```python
from build123d import *

# Parameters (mm, degrees)
BOSS_EXTRUDE1_DEPTH = 19
SKETCH2_W           = 32
SKETCH2_H           = 55
CUT_EXTRUDE1_DEPTH  = 45
SKETCH3_W           = 32
SKETCH3_H           = 22.717187721
CUT_EXTRUDE2_DEPTH  = 12
SKETCH4_R           = 4.5
CUT_EXTRUDE3_DEPTH  = 39
CUT_EXTRUDE4_REACH  = 71
SKETCH5_R           = 5.75
FILLET1_R           = 3


with BuildPart() as part:
    # Sketch1 → Boss-Extrude1 (new body, symmetric)
    with BuildSketch(Plane(origin=(0, 0, 0), x_dir=(0, 0, -1), z_dir=(1, 0, 0))):
        with BuildLine():
            Line((-11, 0), (-11, 58))
            Line((-11, 58), (33, 58))
            Line((33, 58), (10.326710033, -3.789335019))
            ThreePointArc((10.326710033, -3.789335019), (-1.924342697, -10.830369577), (-11, 0))
        make_face()
    extrude(amount=BOSS_EXTRUDE1_DEPTH, both=True)

    # Sketch2 → Cut-Extrude1 (cut, through all)
    with BuildSketch(Plane.XY.offset(11)):
        with Locations((0, 27.5)):
            Rectangle(SKETCH2_W, SKETCH2_H)
    extrude(amount=-CUT_EXTRUDE1_DEPTH, mode=Mode.SUBTRACT)

    # Sketch3 → Cut-Extrude2 (cut, through all)
    with BuildSketch(Plane(origin=(0, 0, 0), x_dir=(1, 0, 0), z_dir=(0, 1, 0))):
        with Locations((0, 0.358593861)):
            Rectangle(SKETCH3_W, SKETCH3_H)
    extrude(amount=-CUT_EXTRUDE2_DEPTH, mode=Mode.SUBTRACT)

    # Sketch4 → Cut-Extrude3 (cut, through all)
    with BuildSketch(Plane.ZY.offset(19)):
        Circle(SKETCH4_R)
    extrude(amount=-CUT_EXTRUDE3_DEPTH, mode=Mode.SUBTRACT)

    # Sketch5 → Cut-Extrude4 (cut, up to next)
    with BuildSketch(Plane(origin=(0, 58, 0), x_dir=(1, 0, 0), z_dir=(0, 1, 0)), mode=Mode.PRIVATE) as cut_extrude4_sk1:
        with Locations((0, 11)):
            Circle(SKETCH5_R)
    cut_extrude4_tool1 = extrude(cut_extrude4_sk1.sketch, amount=-CUT_EXTRUDE4_REACH, mode=Mode.PRIVATE) & part.part
    add(cut_extrude4_tool1.solids().sort_by_distance((0, 58, -11))[0], mode=Mode.SUBTRACT)

    # Fillet1
    fillet1_edges = [part.edges().sort_by_distance(p)[0] for p in [
        (19, 58, -11),
        (-19, 58, -11),
    ]]
    fillet(fillet1_edges, radius=FILLET1_R)


solid = part.part
```
The model under review builds one solid part; all positions refer to its coordinate system, in mm. A direction names the side the tool comes from. Round coordinates to 2 decimals unless told otherwise and drop trailing zeros. Order: outer loops, then holes, each group sorted by start corner. A loop starts at its lowest first (then second) coordinate and runs counter-clockwise, first axis right, second up. Notation, with made-up numbers: (49, -15) -> (86, -15) arc R16 ccw to (86, 5) -> close; hole circle Ø2 at (9.25, 81). An arc over 180 degrees is marked (long way). One line per item, written item: value. Start each with the question number.
Q1. Take a section at A-A (x = 0). Write out the cut boundary in (y, z), and give its area (3 significant figures).
Q2. Machinability: for faces 4 (the face through (4, 58, -6)), 5 (the face through (-4, 55, -5)), which of the approach directions +Z, -Z, +X, -X, +Y, -Y give a long, thin tool a straight path to every point of the face, cutting with its end or side? Answer none if there is none.
Q3. Mouldability with a two-part tool opening along X and no side actions: class faces 1 (the face through (18.14, 57.1, -11.31)), 2 (the face through (16, 29, -5)), 3 (the face through (17.521, -10.866, 1.712)) as released by +X, released by -X, zero draft, split by the parting line, or undercut.
Q4. Take a section at B-B (z = 0). Write out the cut boundary in (x, y).
Q5. Take a section at C-C (y = 16.5). Write out the cut boundary in (x, z).
Q6. Wall thickness on line 1 (X direction, y = 31, z = -9); line 2 (Y direction, x = -6, z = -3.5); line 3 (X direction, y = 55.7, z = -11): over which ranges is each line inside the solid? List them lowest first.
Q7. Clearance check with flat-ended pins moving along their axes: pin 1 Ø2 at (x, z) = (3.5, -28) entering from -Y; pin 2 Ø10 at (x, z) = (15, 6.5) entering from -Y. State where each tip first meets the part, or that it passes through.
Q8. Take a section at D-D (z = -29). Write out the cut boundary in (x, y), and give its area (3 significant figures).
Reported:
1. outline: (55, -31.9) -> (58, -33) -> (58, -16.75) -> (55, -16.75) -> close; (55, -5.25) -> (58, -5.25) -> (58, 11) -> (55, 11) -> close
1. area: 95.8 mm2
2. face 4: +Z, -Z, +X, -X, +Y
2. face 5: +Z, -Z, -Y
3. face 1: released by +X
3. face 2: undercut
3. face 3: zero draft
4. outline: (-19, -11) -> (-16, -11) -> (-16, -4.5) -> (-19, -4.5) -> close; (-19, 4.5) -> (-16, 4.5) -> (-16, 55) -> (16, 55) -> (16, 4.5) -> (19, 4.5) -> (19, 55) arc R3 ccw to (16, 58) -> (-16, 58) arc R3 ccw to (-19, 55) -> close; (16, -11) -> (19, -11) -> (19, -4.5) -> (16, -4.5) -> close
5. outline: (-19, -17.77) -> (-16, -17.77) -> (-16, 11) -> (-19, 11) -> close; (16, -17.77) -> (19, -17.77) -> (19, 11) -> (16, 11) -> close
6. line 1: x = -19 to -16, 16 to 19
6. line 2: y = 55 to 58
6. line 3: x = -18.92 to -5.75, 5.75 to 18.92
7. pin 1: stops at y = 55
7. pin 2: stops at y = -10.88
8. outline: (-19, 47.1) -> (-16, 47.1) -> (-16, 55) -> (16, 55) -> (16, 47.1) -> (19, 47.1) -> (19, 55) arc R3 ccw to (16, 58) -> (-16, 58) arc R3 ccw to (-19, 55) -> close
8. area: 158 mm2
